from build123d import *

# Parameters (mm, degrees)
SKETCH_W          = 6
SKETCH_H          = 15
SKETCH_R          = 1.6
PAD_DEPTH         = 3.5
PAD001_DEPTH      = 1.25
PAD001_DEPTH_BACK = 1.25
CHAMFER_SIZE2     = 2.4
CHAMFER_SIZE      = 3
FILLET_R          = 0.3
FILLET001_R       = 1.5
FILLET002_R       = 1
FILLET003_R       = 0.3


with BuildPart() as part:
    # Sketch (on XY_Plane of Origin) → Pad (new body)
    with BuildSketch(Plane.XY):
        with Locations((7, 0)):
            Rectangle(SKETCH_W, SKETCH_H)
        with Locations((7, 5)):
            Circle(SKETCH_R, mode=Mode.SUBTRACT)
        with Locations((7, -5)):
            Circle(SKETCH_R, mode=Mode.SUBTRACT)
    extrude(amount=-PAD_DEPTH)

    # Sketch003 → Pad001 (join, two sides)
    with BuildSketch(Plane.XZ) as pad001_sk:
        with BuildLine():
            Line((10, 0), (0, 0))
            Line((0, 0), (0, -3.5))
            Line((0, -3.5), (-8, -3.5))
            ThreePointArc((-8, -3.5), (-10.828427, -4.671573), (-12, -7.5))
            Line((-12, -7.5), (-12, -11))
            Line((-12, -11), (-44, -11))
            Line((-44, -11), (-44, -6))
            Line((-44, -6), (-36, -6))
            Line((-36, -6), (-26, 6))
            Line((-26, 6), (10, 6))
            Line((10, 6), (10, 0))
        make_face()
    extrude(amount=PAD001_DEPTH)
    extrude(pad001_sk.sketch, amount=-PAD001_DEPTH_BACK)

    # Chamfer
    chamfer_edges = [part.edges().sort_by_distance(p)[0] for p in [
        (-28, -1.25, -11),
    ]]
    chamfer_side = part.faces().sort_by_distance((-17.427573, -1.25, -2.073781))[0]
    chamfer(chamfer_edges, length=CHAMFER_SIZE, length2=CHAMFER_SIZE2, reference=chamfer_side)

    # Fillet
    fillet_edges = [part.edges().sort_by_distance(p)[0] for p in [
        (-36, 0, -6),
        (-26, 0, 6),
        (0, 0, -3.5),
        (10, 0, 6),
        (0, 0, 0),
    ]]
    fillet(fillet_edges, radius=FILLET_R)

    # Fillet001
    fillet001_edges = [part.edges().sort_by_distance(p)[0] for p in [
        (7, 1.25, 0),
        (7, -1.25, 0),
    ]]
    fillet(fillet001_edges, radius=FILLET001_R)

    # Fillet002
    fillet002_edges = [part.edges().sort_by_distance(p)[0] for p in [
        (4, 1.25, 0.75),
        (4, -1.25, 0.75),
    ]]
    fillet(fillet002_edges, radius=FILLET002_R)

    # Fillet003
    fillet003_edges = [part.edges().sort_by_distance(p)[0] for p in [
        (4, 0, 0),
    ]]
    fillet(fillet003_edges, radius=FILLET003_R)


solid = part.part
Read the model definition and answer for the solid it produces. Units are mm, in the model's axes. A direction names the side the tool comes from. Round coordinates to 2 decimals unless told otherwise and drop trailing zeros. Loops run counter-clockwise (first coordinate to the right, second up) from the corner with the lowest first, then second, coordinate; pieces in that order, holes last. Notation, with made-up numbers: (-23.75, 88) - (12.25, 88) arc R13 ccw to (12.25, 94) - close; hole circle Ø5 at (-22.5, -37.5). An arc over 180 degrees is marked (long way). One line per question, with ' | ' between items. Start each with the question number.
Q1. Section B-B on x = 7 is taken. Give the vertices of the cut face in (y, z).
Q2. Section C-C on x = -38 is taken. Give the vertices of the cut face in (y, z).
Q3. For faces 4 (the flat face through (7, 7.5, -2)), 5 (the flat face through (7, -7, 0)), 6 (the flat face through (-12, 0, -9)), determine the directions among +Z, -Z, +X, -X, +Y, -Y from which every point of the face is accessible in a straight line to the end or side of a thin tool.
Q4. Section A-A on y = -5 is taken. Give the vertices of the cut face in (x, z).
Q5. Find the intervals of material crossed by L1, parallel to Y at x = 7, z = -1.4; L2, parallel to Y at x = -14, z = 4.5; L3, parallel to X at y = -1, z = -2, in increasing order.
Q6. For a pull along X with two mould halves and no side action, classify faces 1 (the flat face through (-17, -1.25, -1)), 2 (the cylindrical face through (5.4, -4.93, -1.73)), 3 (the flat face through (10, 0, -1)) as +X half, -X half, draft (parallel to the pull), parting line (faces both ways), or undercut.
Q7. Section D-D on z = -9.5 is taken. Give the vertices of the cut face in (x, y), plus the area to 3 significant figures.
Q8. Flat-ended cylindrical pins translate along their axes: pin 1 (2 mm diameter, centred on x = -30.5, y = 0.5, fed in from +Z); pin 2 (2.5 mm diameter, centred on x = 5.5, y = 5, fed in from +Z); pin 3 (0.8 mm diameter, centred on x = -3, y = 0, fed in from -Z). Find the tip coordinate at first contact, or state that the pin passes through.
Established:
1) outline: (-7.5, -3.5) - (-6.6, -3.5) - (-6.6, 0) - (-7.5, 0) - close; (-3.4, -3.5) - (3.4, -3.5) - (3.4, 0) - (2.75, 0) arc R1.5 cw to (1.25, 1.5) - (1.25, 6) - (-1.25, 6) - (-1.25, 1.5) arc R1.5 cw to (-2.75, 0) - (-3.4, 0) - close; (6.6, -3.5) - (7.5, -3.5) - (7.5, 0) - (6.6, 0) - close
2) outline: (-1.25, -8) - (1.15, -11) - (1.25, -11) - (1.25, -6) - (-1.25, -6) - close
3) face 4: +Z, -Z, +X, -X, +Y | face 5: +Z, +X, -X, -Y | face 6: -Z, +X, +Y, -Y
4) outline: (4, -3.5) - (5.4, -3.5) - (5.4, 0) - (4, 0) - close; (8.6, -3.5) - (10, -3.5) - (10, 0) - (8.6, 0) - close
5) L1: -7.5 to -6.6, -3.4 to 3.4, 6.6 to 7.5 | L2: -1.25 to 1.25 | L3: -32.67 to 0, 4 to 10
6) face 1: draft | face 2: undercut | face 3: +X half
7) outline: (-44, -0.05) - (-12, -0.05) - (-12, 1.25) - (-44, 1.25) - close | area: 41.6 mm²
8) pin 1: z = 1.8 | pin 2: z = 0 | pin 3: z = -3.5
